from build123d import *

# Parameters (mm, degrees)
F0_W     = 10
F0_H     = 30
F0_W_2   = 8
F0_H_2   = 15
F0_R     = 17.5
F1_DEPTH = 15


with BuildPart() as f1:
    # F0 (on Top) → F1 (new body)
    with BuildSketch(Plane.XY):
        Polygon((-13.852531, 0), (-13.852531, 25), (-168.852531, 25), (-168.852531, 0), (-158.852531, 0), (-148.852531, 0), (-140.852531, 0), (-130.852531, 0), (-123.852531, 0), (-116.852531, 0), align=None)
        with Locations((-163.852531, -15)):
            Rectangle(F0_W, F0_H)
        with Locations((-144.852531, -7.5)):
            Rectangle(F0_W_2, F0_H_2)
        Polygon((-123.852531, -15.00006), (-123.852531, 0), (-130.852531, 0), align=None)
        Polygon((-123.852531, -15.00006), (-116.852531, 0), (-123.852531, 0), align=None)
        with BuildLine():
            ThreePointArc((-13.852531, 0), (53.839211, 12.5), (-13.852531, 25))
            Line((-13.852531, 25), (-13.852531, 0))
        make_face()
        with Locations((18.839211, 12.5)):
            Circle(F0_R, mode=Mode.SUBTRACT)
        with Locations((18.839211, 12.5)):
            Circle(F0_R)
    extrude(amount=F1_DEPTH)


solid = f1.part
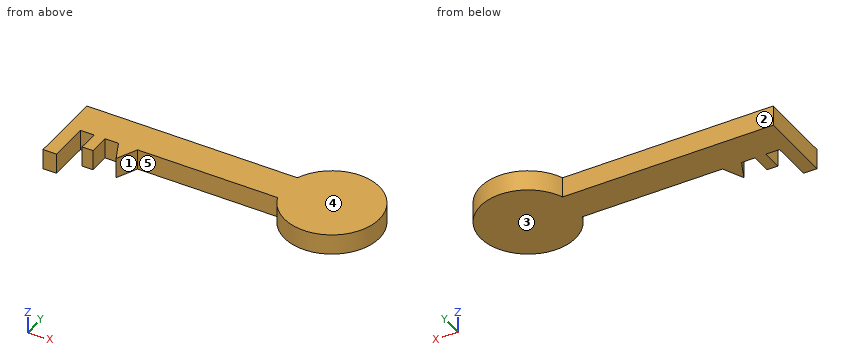
CAD build for the part. Positions are in the model's coordinates, mm. Face numbers are marked on the shaded views. A direction names the side the tool comes from. Round coordinates to 2 decimals unless told otherwise and drop trailing zeros. Write each loop counter-clockwise with the first axis right and the second up, starting at its lowest first coordinate (ties: lowest second). Pieces come first, ordered by that corner, then holes. Notation, with made-up numbers: M 57,-2.75 L 106,-2.75 A13 cw 106,17.25 Z; hole C -25.5,47.25 d10. An arc over 180 degrees is marked long. Use a Markdown table: item, result. Add a question column.
1. Pull direction X, two halves, no side cores. Call the marked faces 4 and 5: released by +X, released by -X, zero draft, split by the parting line, or undercut.
2. Drill centre lines: probe 1 along X at (y, z) = (-14, 12); probe 2 along X at (y, z) = (-0.5, 4.5); probe 3 along Y at (x, z) = (-55, 2.5). Where is each one in solid material? Low to high.
3. Slice it at C-C on x = -61.5. Give the cut face in (y, z), then the cut area to 3 significant figures.
4. Slice it at B-B on z = 11.5. Give the cut face in (x, y).
5. 3-axis set-ups, long thin cutter, end or side, ignore diameter. For the marked faces 1, 2 and 3: which of +Z, -Z, +X, -X, +Y, -Y reach the whole face in a straight line?
6. Flat gauge pins, fed straight in: P1, Ø5, axis at x = -137, z = 8, coming from the -Y side; P2, Ø6.5, axis at x = -145.5, z = 7.5, coming from the -Y side; P3, Ø2, axis at y = -15.5, z = 13.5, coming from the +X side; P4, Ø5, axis at x = 14, y = -0.5, coming from the -Z side. Where does each tip first touch, or does it go through?
7. Slice it at A-A on y = -9. Give the cut face in (x, z), then the cut area to 3 significant figures.
Reply:
| question | item | result |
|---|---|---|
| 1 | face 4 | zero draft |
| 1 | face 5 | undercut |
| 2 | probe 1 | x = -168.85 to -158.85, -148.85 to -140.85, -124.32 to -123.39, -4.02 to 41.7 |
| 2 | probe 2 | x = -168.85 to -158.85, -148.85 to -140.85, -130.62 to -117.09, -13.66 to 51.34 |
| 2 | probe 3 | y = 0 to 25 |
| 3 | outline | M 0,0 L 25,0 L 25,15 L 0,15 Z |
| 3 | area | 375 mm^2 |
| 4 | outline | M -168.85,-30 L -158.85,-30 L -158.85,0 L -148.85,0 L -148.85,-15 L -140.85,-15 L -140.85,0 L -130.85,0 L -123.85,-15 L -116.85,0 L -13.85,0 A35 ccw long -13.85,25 L -168.85,25 Z |
| 5 | face 1 | +Z, -Z, -Y |
| 5 | face 2 | +Z, -Z, -X, +Y |
| 5 | face 3 | -Z, +X, -X, +Y, -Y |
| 6 | P1 | stops at y = 0 |
| 6 | P2 | stops at y = -15 |
| 6 | P3 | stops at x = 41.11 |
| 6 | P4 | stops at z = 0 |
| 7 | outline | M -168.85,0 L -158.85,0 L -158.85,15 L -168.85,15 Z; M -148.85,0 L -140.85,0 L -140.85,15 L -148.85,15 Z; M -126.65,0 L -121.05,0 L -121.05,15 L -126.65,15 Z; M -8.78,0 L 46.46,0 L 46.46,15 L -8.78,15 Z |
| 7 | area | 1,180 mm^2 |
